Input: part model. Units: mm. Frame: model coordinates. A direction names the side the tool comes from. Give positions to 0.01 mm unless a question says otherwise; leave off trailing zeros. Loops run counter-clockwise (first coordinate to the right, second up) from the corner with the lowest first, then second, coordinate; pieces in that order, holes last.
Autodesk Inventor part; units mm, degrees
ref_plane "YZ Plane" through (0, 0, 0) normal (1, 0, 0) x (0, 1, 0)
ref_plane "XZ Plane" through (0, 0, 0) normal (0, 1, 0) x (-1, 0, 0)
ref_plane "XY Plane" through (0, 0, 0) normal (0, 0, 1) x (1, 0, 0)
sketch "Sketch1" plane through (0, 0, 0) normal (0, 0, 1) x (1, 0, 0)
  line L0 (0, 0) -> (22, 0)
  line L1 (22, 0) -> (22, -9.2)
  line L2 (22, -9.2) -> (0, -9.2)
  line L3 (0, -9.2) -> (0, 0)
  dimension "d0" = 22
  dimension "d1" = 9.2
extrude "Extrusion1" add sketch "Sketch1" along normal blind 9.2
sketch "Sketch2" plane through (0, 0, 9.2) normal (0, 0, 1) x (1, 0, 0)
  line L0 (0.9024, -0.8915) -> (20.9524, -0.8915)
  line L1 (20.9524, -0.8915) -> (20.9524, -8.0915)
  line L2 (20.9524, -8.0915) -> (0.9024, -8.0915)
  line L3 (0.9024, -8.0915) -> (0.9024, -0.8915)
  point P0 (0, 0)
  dimension "d4" = 20.05
  dimension "d5" = 7.2
extrude "Extrusion2" cut sketch "Sketch2" against normal blind 7.2
sketch "Sketch3" plane through (0, 0, 0) normal (0, 0, -1) x (-1, 0, 0)
  circle A0 centre (-10.8985, -4.6543) radius 1.435
  point P0 (0, 0)
  dimension "d8" = 2.87
extrude "Extrusion3" cut sketch "Sketch3" against normal blind 7.2
properties part number "Fader Cap"
(1) Cut plane A-A (z = 6.5). Return the cut outline in (x, y), and give its area (3 significant figures).
Values follow:
outline: (0, -9.2) - (22, -9.2) - (22, 0) - (0, 0) - close; hole (0.9, -8.09) - (20.95, -8.09) - (20.95, -0.89) - (0.9, -0.89) - close
area: 58.0 mm2
(2) Mould query, pull axis Y, two halves, no side actions, for faces 1 (the flat face through (11, -0.892, 6)), 2 (the flat face through (11, 0, 5)), 3 (the flat face through (0, -5, 5)). Classes: +Y half, -Y half, draft (parallel to the pull), parting line (faces both ways), or undercut.
Values follow:
face 1: undercut
face 2: +Y half
face 3: draft
(3) Cut plane B-B (x = 14). Return the cut outline in (y, z), and give its area (3 significant figures).
Values follow:
outline: (-9.2, 0) - (0, 0) - (0, 9.2) - (-0.89, 9.2) - (-0.89, 2) - (-8.09, 2) - (-8.09, 9.2) - (-9.2, 9.2) - close
area: 32.8 mm2
(4) Pin query (flat end, axial travel): pin 1 Ø1 at (x, y) = (8.5, -2.5) entering from +Z; pin 2 Ø1.7 at (x, y) = (10.9, -4.65) entering from -Z. Return the tip coordinate at first contact, or that it passes through.
Values follow:
pin 1: stops at z = 2
pin 2: passes through
(5) Reachability of faces 4 (the flat face through (11, -3, 2)), 5 (the flat face through (11, -9.2, 5)) from +Z, -Z, +X, -X, +Y, -Y: full face, straight path, thin tool, end or side. Return the list, or none.
Values follow:
face 4: +Z
face 5: +Z, -Z, +X, -X, -Y
(6) Cut plane D-D (y = -7). Return the cut outline in (x, z).
Values follow:
outline: (0, 0) - (22, 0) - (22, 9.2) - (20.95, 9.2) - (20.95, 2) - (0.9, 2) - (0.9, 9.2) - (0, 9.2) - close
(7) Ray query, probe 1 along X at (y, z) = (-2, 5.25); probe 2 along Y at (x, z) = (13, 2.75); probe 3 along Z at (x, y) = (8, -3.5). Return the intervals inside material, ascending.
Values follow:
probe 1: x = 0 to 0.9, 20.95 to 22
probe 2: y = -9.2 to -8.09, -0.89 to 0
probe 3: z = 0 to 2
(8) Cut plane C-C (y = -3.5). Return the cut outline in (x, z), and give its area (3 significant figures).
Values follow:
outline: (0, 0) - (10.05, 0) - (10.05, 2) - (0.9, 2) - (0.9, 9.2) - (0, 9.2) - close; (11.75, 0) - (22, 0) - (22, 9.2) - (20.95, 9.2) - (20.95, 2) - (11.75, 2) - close
area: 54.6 mm2
